For this review, use the dimensioned drawing (mm, ordinates from the lowest corner) and the shaded views. A direction names the side the tool comes from. Coordinates: 2 decimals unless noted, no trailing zeros. Loops run counter-clockwise (first coordinate to the right, second up) from the corner with the lowest first, then second, coordinate; pieces in that order, holes last. Notation, with made-up numbers: M 36.25,46 L 85.25,46 A15 ccw 85.25,61 Z; hole C 65.5,18.25 d3. An arc over 180 degrees is marked long. Write each question's results on one line, items separated by ' | '. Start each with the question number.
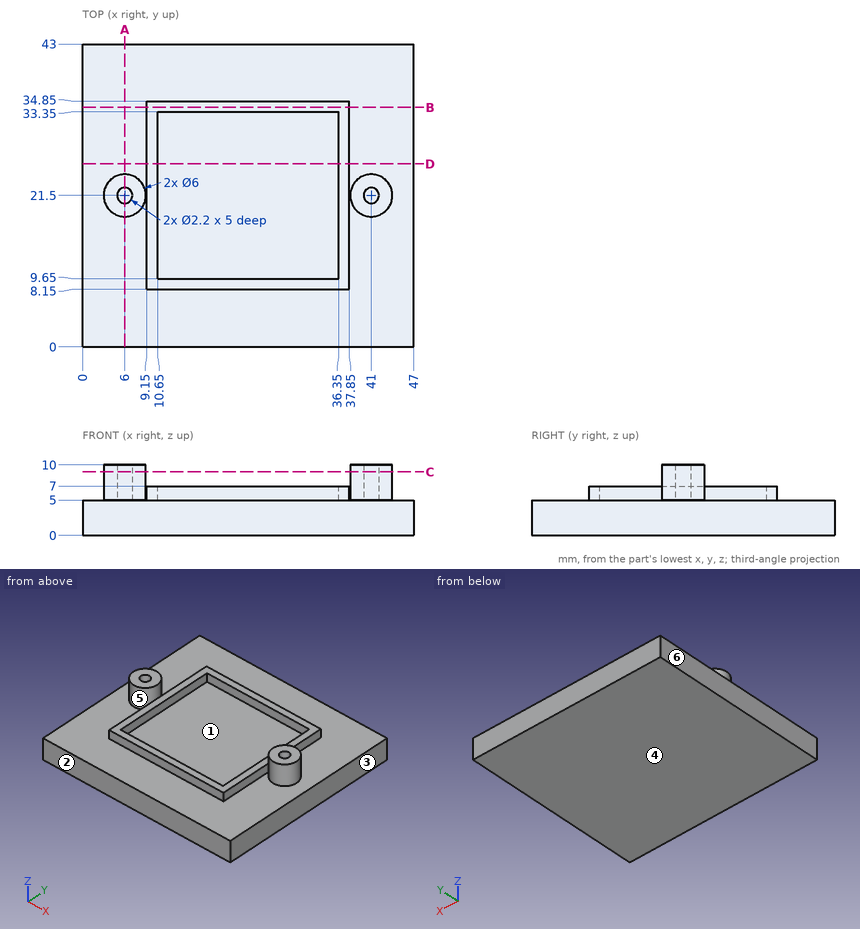
Q1. To check wall thickness, follow line 1 along Y through (x, z) = (6, 8); line 2 along Z through (x, y) = (19, 10.5); line 3 along Y through (x, z) = (19.5, 5.25). State the ranges of each line that lie inside material, in increasing order.
Q2. Take a section at D-D, the plane y = 26. Give the boundary of the cut face in (x, z), then the cut area to 3 significant figures.
Q3. Take a section at C-C, the plane z = 9. Give the boundary of the cut face in (x, y), then the cut area to 3 significant figures.
Q4. The part is to be moulded in two halves that separate along X. For the marked faces 3, 4, 5 and 6, say which applies: pulls with the +X half, pulls with the -X half, needs draft (parallel to the pull), parting line crosses it, or undercut.
Q5. Take a section at A-A, the plane x = 6. Give the boundary of the cut face in (y, z), then the cut area to 3 significant figures.
Q6. Insertion check: P1, Ø1, axis at x = 29.5, z = 6.5, coming from the -Y side; P2, Ø12, axis at x = 25, y = 25, coming from the +Z side; P3, Ø0.6, axis at y = 26.5, z = 6.5, coming from the +X side. Each pin has a flat end and moves straight along its axis. Give the tip position at first contact, or say it passes through.
Q7. For the marked faces 1 and 2, list the 3-axis set-ups (+Z, -Z, +X, -X, +Y, -Y) from which the entire face can be reached by the end or side of a thin tool; tool diameter is ignored.
Q8. Take a section at B-B, the plane y = 34. Give the boundary of the cut face in (x, z), then the cut area to 3 significant figures.
Results:
1) line 1: 18.5 to 20.4, 22.6 to 24.5 | line 2: 0 to 5 | line 3: 8.15 to 9.65, 33.35 to 34.85
2) outline: M 0,0 L 47,0 L 47,5 L 37.85,5 L 37.85,7 L 36.35,7 L 36.35,5 L 10.65,5 L 10.65,7 L 9.15,7 L 9.15,5 L 0,5 Z | area: 241 mm^2
3) outline: C 6,21.5 d6; C 41,21.5 d6; hole C 6,21.5 d2.2; hole C 41,21.5 d2.2 | area: 48.9 mm^2
4) face 3: pulls with the +X half | face 4: needs draft | face 5: undercut | face 6: pulls with the -X half
5) outline: M 0,0 L 43,0 L 43,5 L 24.5,5 L 24.5,10 L 22.6,10 L 22.6,5 L 20.4,5 L 20.4,10 L 18.5,10 L 18.5,5 L 0,5 Z | area: 234 mm^2
6) P1: y = 8.15 | P2: z = 5 | P3: x = 37.85
7) face 1: +Z | face 2: +Z, -Z, +X, -X, -Y
8) outline: M 0,0 L 47,0 L 47,5 L 37.85,5 L 37.85,7 L 9.15,7 L 9.15,5 L 0,5 Z | area: 292 mm^2
